Input: dimensioned drawing with shaded views. Units: mm. Origin: part minimum x, y, z. A direction names the side the tool comes from. Round coordinates to 2 decimals unless told otherwise and drop trailing zeros. Write each loop counter-clockwise with the first axis right and the second up, starting at its lowest first coordinate (ties: lowest second). Pieces come first, ordered by that corner, then holes. Notation, with made-up numbers: M 36.25,45 L 93.25,45 A34 cw 93.25,81 Z; hole C 47,-23.5 d11. An arc over 180 degrees is marked long. Use one line per item in the form item = value. Start each with the question number.
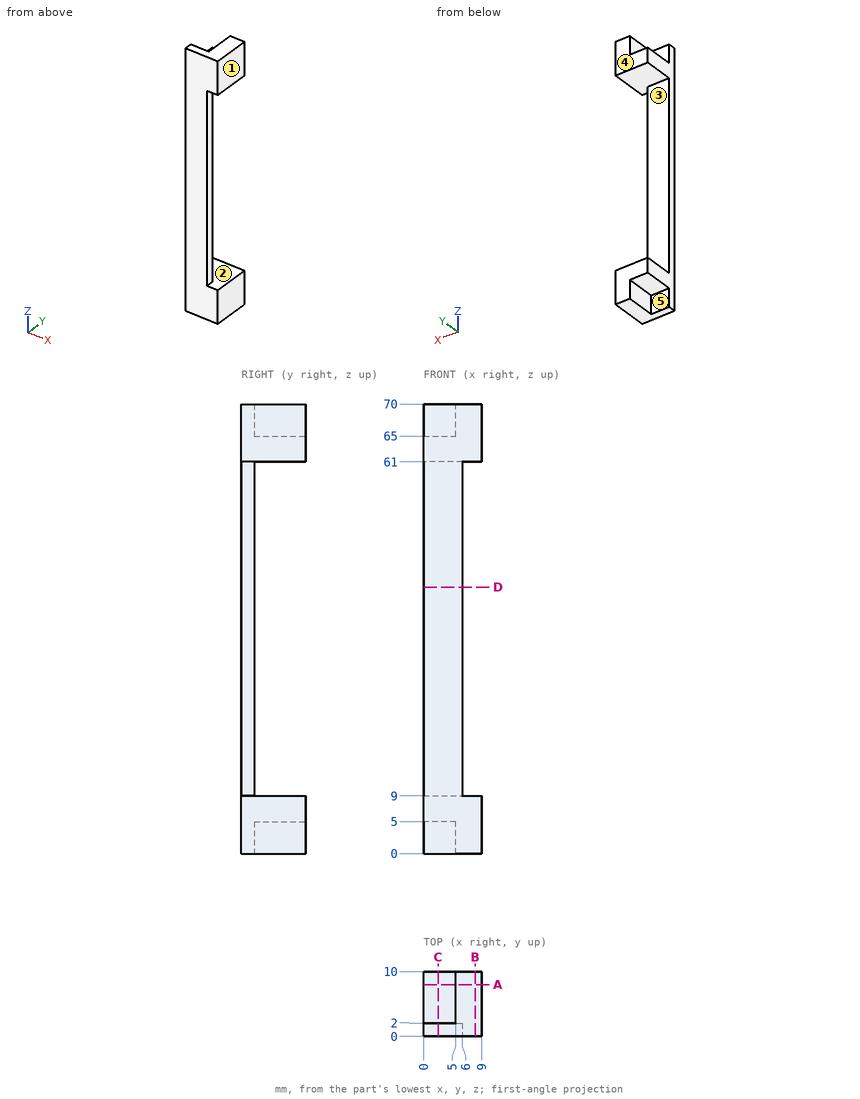
1. Section query A-A (y = 8). Return loops of the section in (x, z), then the cut area to 3 significant figures.
2. Ray query, probe 1 along Z at (x, y) = (1.5, 3.5); probe 2 along Z at (x, y) = (8.75, 5); probe 3 along X at (y, z) = (0.75, 38). Return the intervals inside material, ascending.
3. Section query B-B (x = 8). Return loops of the section in (y, z).
4. Contact query for flat-ended pins moving along their axis: pin 1 (3 mm diameter, centred on x = 4, z = 32.5, fed in from +Y); pin 2 (1.5 mm diameter, centred on x = 1, y = 3.5, fed in from -Z); pin 3 (1.6 mm diameter, centred on y = 1, z = 38.5, fed in from +X). Output: stop coordinate, or through.
5. Set-up query: the marked faces 3, 4 and 5. Return all of +Z, -Z, +X, -X, +Y, -Y with unobstructed straight access to the full face (end or side cutting, diameter ignored); none if empty.
6. Section query D-D (z = 41.5). Return loops of the section in (x, y), then the cut area to 3 significant figures.
7. Pull-direction query (Z, two-part tool) for the marked faces 1 and 2; classes: released by +Z, released by -Z, zero draft, split by the parting line, or undercut.
8. Section query C-C (x = 2.25). Return loops of the section in (y, z).
Checks:
q1.outline = M 0,5 L 5,5 L 5,0 L 9,0 L 9,9 L 0,9 Z; M 0,61 L 9,61 L 9,70 L 5,70 L 5,65 L 0,65 Z
q1.area = 112 mm^2
q2.probe_1 = 5 to 9, 61 to 65
q2.probe_2 = 0 to 9, 61 to 70
q2.probe_3 = 0 to 6
q3.outline = M 0,0 L 10,0 L 10,9 L 0,9 Z; M 0,61 L 10,61 L 10,70 L 0,70 Z
q4.pin_1 = 2
q4.pin_2 = 5
q4.pin_3 = 6
q5.face_3 = +X, -X, +Y
q5.face_4 = +Z, -Z, +X, -X, +Y
q5.face_5 = -Z, -X, +Y
q6.outline = M 0,0 L 6,0 L 6,2 L 0,2 Z
q6.area = 12.0 mm^2
q7.face_1 = zero draft
q7.face_2 = undercut
q8.outline = M 0,0 L 2,0 L 2,5 L 10,5 L 10,9 L 2,9 L 2,61 L 10,61 L 10,65 L 2,65 L 2,70 L 0,70 Z
